Check sheet for the modelled part. Datum: model origin and axes. Units: mm. A direction names the side the tool comes from. Coordinates: 2 decimals unless noted, no trailing zeros. Write each loop counter-clockwise with the first axis right and the second up, starting at its lowest first coordinate (ties: lowest second). Pieces come first, ordered by that corner, then holes. Notation, with made-up numbers: (-21, 33) - (-1, 33) arc R10 ccw to (-1, 38) - close; hole circle Ø4 at (48, -2). An arc over 180 degrees is marked (long way). Use one line per item in the form item = value. Start each with the question number.
1. Cross-section at C-C on y = -5.5. Record the boundary of the cut face in (x, z), then the cut area to 3 significant figures.
2. Scan lines: line 1 along Z through (x, y) = (0, 8.5); line 2 along Y through (x, z) = (36.5, 0); line 3 along X through (y, z) = (68, 0). Record each from-to range of solid material in increasing order.
3. Cross-section at B-B on x = 0. Record the boundary of the cut face in (y, z), then the cut area to 3 significant figures.
4. Cross-section at D-D on x = 52. Record the boundary of the cut face in (y, z), then the cut area to 3 significant figures.
5. Cross-section at A-A on z = 0. Record the boundary of the cut face in (x, y).
6. Go/stop test with flat-tipped pins: pin 1 Ø1 at (x, z) = (-21.5, -9) entering from +Y; pin 2 Ø10 at (y, z) = (69.5, 5.5) entering from -X; pin 3 Ø6 at (y, z) = (52.5, -3.5) entering from +X. Record where each tip stops, or that it passes through.
7. Tool access check on faces 5 (the face through (0.638, 63.668, -14.486)), 6 (the face through (3.1, 120, -11.1)). Record the directions out of +Z, -Z, +X, -X, +Y, -Y that give a thin tool (end or side, any length) a straight path to the whole face; none if there is none.
8. Draft check along Z on faces 1 (the face through (63, 13.1, 1.3)), 2 (the face through (-0.88, -15.62, -3.47)), 3 (the face through (-0.88, -12.69, -2.82)), 4 (the face through (-0.572, 11.435, 12.987)). Enter one of: +Z half, -Z half, draft (parallel to the pull), parting line (faces both ways), or undercut.
```python
from build123d import *

# Parameters (mm, degrees)
SKETCH1_W                = 126
SKETCH1_H                = 16
M22_CLEARANCE_HOLE1_D    = 26
BOSS_EXTRUDE1_REACH      = 152.735
BOSS_EXTRUDE1_END_RADIUS = 16
SKETCH4_R                = 14.5
CUT_EXTRUDE1_REACH       = 122.529
CUT_EXTRUDE1_END_RADIUS  = 13
SKETCH5_R                = 13
SKETCH6_R                = 9.097381441
CUT_EXTRUDE2_DEPTH       = 0.4
CUT_EXTRUDE2_DRAFT       = -70
SKETCH7_R                = 7.998390473
CUT_EXTRUDE3_DEPTH       = 1.26
CUT_EXTRUDE3_DRAFT       = 50
SKETCH8_R                = 9.5
CUT_EXTRUDE4_DEPTH       = 30.5245
SKETCH9_R                = 11.3155
CUT_EXTRUDE5_DEPTH       = 119.8155
CHAMFER1_SIZE            = 1
FILLET1_R                = 3.2


with BuildPart() as part:
    # Sketch1 → Revolve1 (revolve)
    with BuildSketch(Plane(origin=(0, 0, 0), x_dir=(-1, 0, 0), z_dir=(0, 0, -1)), mode=Mode.PRIVATE) as revolve1_sk:
        with Locations((0, 8)):
            Rectangle(SKETCH1_W, SKETCH1_H)
    revolve(revolve1_sk.sketch.rotate(Axis((63, 0, 0), (-1, 0, 0)), 270), axis=Axis((63, 0, 0), (-1, 0, 0)))

    # M22 Clearance Hole1 (through all)
    with Locations(Plane(origin=(63, 0, 0), x_dir=(0, 0, -1), z_dir=(1, 0, 0))):
        with Locations((0, 0)):
            Hole(M22_CLEARANCE_HOLE1_D / 2)

    # Boss-Extrude1: up to this cylinder (the profile starts outside it)
    boss_extrude1_end = Plane(origin=(0, 0, 0), z_dir=(-1, 0, 0)) * Cylinder(BOSS_EXTRUDE1_END_RADIUS, 338.47, mode=Mode.PRIVATE)
    # Sketch4 → Boss-Extrude1 (add, up to the surface)
    with BuildSketch(Plane(origin=(0, 120, 0), x_dir=(1, 0, 0), z_dir=(0, 1, 0)), mode=Mode.PRIVATE) as boss_extrude1_sk1:
        with Locations(Location((0, 0, 0), (0, 0, 270))):
            Circle(SKETCH4_R)
    boss_extrude1_tool1 = extrude(boss_extrude1_sk1.sketch, amount=-BOSS_EXTRUDE1_REACH, mode=Mode.PRIVATE) - boss_extrude1_end
    add(boss_extrude1_tool1.solids().sort_by_distance((0, 120, 0))[0])

    # Cut-Extrude1: up to this cylinder (the profile starts outside it)
    cut_extrude1_end = Plane(origin=(0, 0, 0), z_dir=(1, 0, 0)) * Cylinder(CUT_EXTRUDE1_END_RADIUS, 272.058, mode=Mode.PRIVATE)
    # Sketch5 → Cut-Extrude1 (cut, up to the surface)
    with BuildSketch(Plane(origin=(0, 18.5, 0), x_dir=(1, 0, 0), z_dir=(0, 1, 0)), mode=Mode.PRIVATE) as cut_extrude1_sk1:
        with Locations(Location((0, 0, 0), (0, 0, 90))):
            Circle(SKETCH5_R)
    cut_extrude1_tool1 = extrude(cut_extrude1_sk1.sketch, amount=-CUT_EXTRUDE1_REACH, mode=Mode.PRIVATE) - cut_extrude1_end
    add(cut_extrude1_tool1.solids().sort_by_distance((0, 18.5, 0))[0], mode=Mode.SUBTRACT)


with BuildPart() as cut_extrude2_tool:
    # Sketch6 → Cut-Extrude2 (with draft: the straight prism first)
    with BuildSketch(Plane.XZ.offset(-18.5)):
        Circle(SKETCH6_R)
    extrude(amount=-CUT_EXTRUDE2_DEPTH)
    # Cut-Extrude2: the draft: its side faces are tilted about the plane it starts from
    cut_extrude2_sides = [cut_extrude2_tool.faces().sort_by_distance(p)[0] for p in [
        (-9.097381441, 18.7, 0),
    ]]
    draft(cut_extrude2_sides, Plane.XZ.offset(-18.5), CUT_EXTRUDE2_DRAFT)


with BuildPart() as part_1:
    add(part.part)

    # Cut-Extrude2: cut by cut_extrude2_tool
    add(cut_extrude2_tool.part, mode=Mode.SUBTRACT)


with BuildPart() as cut_extrude3_tool:
    # Sketch7 → Cut-Extrude3 (with draft: the straight prism first)
    with BuildSketch(Plane.XZ.offset(-18.9)):
        Circle(SKETCH7_R)
    extrude(amount=-CUT_EXTRUDE3_DEPTH)
    # Cut-Extrude3: the draft: its side faces are tilted about the plane it starts from
    cut_extrude3_sides = [cut_extrude3_tool.faces().sort_by_distance(p)[0] for p in [
        (-7.998390473, 19.53, 0),
    ]]
    draft(cut_extrude3_sides, Plane.XZ.offset(-18.9), CUT_EXTRUDE3_DRAFT)


with BuildPart() as part_2:
    add(part_1.part)

    # Cut-Extrude3: cut by cut_extrude3_tool
    add(cut_extrude3_tool.part, mode=Mode.SUBTRACT)

    # Sketch8 → Cut-Extrude4 (cut)
    with BuildSketch(Plane.XZ.offset(-20.16)):
        with Locations(Location((0, 0, 0), (0, 0, 90))):
            Circle(SKETCH8_R)
    extrude(amount=-CUT_EXTRUDE4_DEPTH, mode=Mode.SUBTRACT)

    # Sketch9 → Cut-Extrude5 (cut)
    with BuildSketch(Plane(origin=(0, 120, 0), x_dir=(-1, 0, 0), z_dir=(0, 1, 0))):
        with Locations(Location((0, 0, 0), (0, 0, 270))):
            Circle(SKETCH9_R)
    extrude(amount=-CUT_EXTRUDE5_DEPTH, mode=Mode.SUBTRACT)

    # Chamfer1
    chamfer1_edges = [part_2.edges().sort_by_distance(p)[0] for p in [
        (0, 120, -14.5),
    ]]
    chamfer(chamfer1_edges, length=CHAMFER1_SIZE)

    # Fillet1
    # the kernel refuses this fillet: 3.2 mm, written as the material it adds along each edge
    with BuildSketch(Plane(origin=(0, 18.5, 0), x_dir=(0, 0, -1), z_dir=(1, 0, 0))) as fillet1_piece_1:
        with BuildLine():
            CenterArc((9.8, -2.818378922), FILLET1_R, 0, 61.73217134)
            Line((13, -2.818378922), (13.064, -2.818378922))
            Line((13.064, -2.818378922), (13.064, 0))
            Line((13.064, 0), (13, 0.064))
            ThreePointArc((13, 0.064), (12.15775, 0.064), (11.34581, 0.056367578))
            Line((11.34581, 0.056367578), (11.3155, 0))
        make_face()
    revolve(axis=Axis((0, 18.5, 0), (0, 1, 0)))


solid = part_2.part
```
Final values:
q1.outline = (-63, -15.02) - (63, -15.02) - (63, -11.78) - (-63, -11.78) - close; (-63, 11.78) - (63, 11.78) - (63, 15.02) - (-63, 15.02) - close
q1.area = 818 mm²
q2.line_1 = -14.5 to -13, 13 to 14.5
q2.line_2 = -16 to -13, 13 to 16
q2.line_3 = -14.5 to -11.32, 11.32 to 14.5
q3.outline = (0, -13) arc R13 cw to (0, 13) - (15.68, 13) arc R3.2 cw to (18.5, 11.32) - (120, 11.32) - (120, 13.5) - (119, 14.5) - (6.76, 14.5) arc R16 ccw (long way) to (6.76, -14.5) - (119, -14.5) - (120, -13.5) - (120, -11.32) - (18.5, -11.32) arc R3.2 cw to (15.68, -13) - close
q3.area = 854 mm²
q4.outline = circle Ø32 at (0, 0); hole circle Ø26 at (0, 0)
q4.area = 273 mm²
q5.outline = (-63, -16) - (63, -16) - (63, -13) - (-63, -13) - close; (-63, 13) - (-13, 13) - (-13, 15.68) arc R3.2 cw to (-11.32, 18.5) - (-11.32, 120) - (-13.5, 120) - (-14.5, 119) - (-14.5, 16) - (-63, 16) - close; (11.32, 18.5) arc R3.2 cw to (13, 15.68) - (13, 13) - (63, 13) - (63, 16) - (14.5, 16) - (14.5, 119) - (13.5, 120) - (11.32, 120) - close
q6.pin_1 = 13.56
q6.pin_2 = -14.49
q6.pin_3 = 14.49
q7.face_5 = +Y
q7.face_6 = +Z, -Z, +X, -X, +Y
q8.face_1 = draft
q8.face_2 = parting line
q8.face_3 = undercut
q8.face_4 = undercut
